Here's how the part is built. I have some questions about the finished solid (model axes, mm). Round coordinates to 2 decimals unless told otherwise and drop trailing zeros. Answer as CSV lines item,"result".
```python
from build123d import *

# Parameters (mm, degrees)
ESQUISSE1_W             = 424
ESQUISSE1_H             = 503
BOSS_EXTRU_1_DEPTH      = 10
ENL_V_MAT_EXTRU_1_DEPTH = 5
CHANFREIN1_SIZE         = 5


with BuildPart() as part:
    # Esquisse1 → Boss.-Extru.1 (new body)
    with BuildSketch(Plane.XY):
        with Locations((212, 251.5)):
            Rectangle(ESQUISSE1_W, ESQUISSE1_H)
    extrude(amount=BOSS_EXTRU_1_DEPTH)

    # Esquisse2 → Enlèv. mat.-Extru.1 (cut)
    with BuildSketch(Plane.XY.offset(10)):
        Polygon((100, 231.923881554), (100, 271.076118446), (40, 331.076118446), (40, 171.923881554), align=None)
        Polygon((191.923881554, 363), (232.076118446, 363), (332.076118446, 463), (91.923881554, 463), align=None)
        Polygon((40, 463), (40, 373.502525317), (130, 283.502525317), (130, 219.497474683), (40, 129.497474683), (40, 40), (49.497474683, 40), (179.497474683, 170), (244.502525317, 170), (374.502525317, 40), (384, 40), (384, 129.497474683), (294, 219.497474683), (294, 283.502525317), (384, 373.502525317), (384, 463), (374.502525317, 463), (244.502525317, 333), (179.497474683, 333), (49.497474683, 463), align=None)
        Polygon((324, 231.923881554), (324, 271.076118446), (384, 331.076118446), (384, 171.923881554), align=None)
        Polygon((332.076118446, 40), (91.923881554, 40), (191.923881554, 140), (232.076118446, 140), align=None)
    extrude(amount=-ENL_V_MAT_EXTRU_1_DEPTH, mode=Mode.SUBTRACT)

    # Chanfrein1
    chanfrein1_edges = [part.edges().sort_by_distance(p)[0] for p in [
        (212, 40, 5),
        (141.923881554, 90, 5),
        (212, 140, 5),
        (282.076118446, 90, 5),
        (40, 251.5, 5),
        (70, 301.076118446, 5),
        (100, 251.5, 5),
        (70, 201.923881554, 5),
        (384, 251.5, 5),
        (354, 201.923881554, 5),
        (324, 251.5, 5),
        (354, 301.076118446, 5),
        (114.497474683, 398, 5),
        (212, 333, 5),
        (309.502525317, 398, 5),
        (379.251262658, 463, 5),
        (384, 418.251262658, 5),
        (339, 328.502525317, 5),
        (294, 251.5, 5),
        (339, 174.497474683, 5),
        (384, 84.748737342, 5),
        (379.251262658, 40, 5),
        (309.502525317, 105, 5),
        (212, 170, 5),
        (114.497474683, 105, 5),
        (44.748737342, 40, 5),
        (40, 84.748737342, 5),
        (85, 174.497474683, 5),
        (130, 251.5, 5),
        (85, 328.502525317, 5),
        (40, 418.251262658, 5),
        (44.748737342, 463, 5),
        (212, 463, 5),
        (282.076118446, 413, 5),
        (212, 363, 5),
        (141.923881554, 413, 5),
    ]]
    chamfer(chanfrein1_edges, length=CHANFREIN1_SIZE - 0.0001)  # a hair under: the kernel refuses the full size


solid = part.part
```
1. For pin 1 Ø1.5 at (y, z) = (273, 2.5) entering from -X, with a flat end and sliding along its axis, tell me the tip position at first contact or that it passes through.
Numbers:
pin 1,"stops at x = 0"
2. If I drill on line 1 (Y direction, x = 49, z = 9.5); line 2 (X direction, y = 50.5, z = 9.5); line 3 (X direction, y = 143.5, z = 7), over which ranges is the centre line in solid material (lowest first)?
Numbers:
line 1,"y = 0 to 40.5, 137.79 to 181.63, 321.37 to 365.21, 462.5 to 503"
line 2,"x = 0 to 40.5, 59.29 to 103.13, 320.87 to 364.71, 383.5 to 424"
line 3,"x = 0 to 58.25, 148.75 to 275.25, 365.75 to 424"
3. If we mould it in two halves opening along X, with no side actions, what happens to faces 1 (the face through (424, 248, 5)), 2 (the face through (311.483, 396.396, 7.465))? For each: released by +X, released by -X, zero draft, split by the parting line, or undercut.
Numbers:
face 1,"released by +X"
face 2,"undercut"
